```python
from build123d import *

# Parameters (mm, degrees)
ESQUISSE1_W                                        = 10
ESQUISSE1_H                                        = 10
BOSS_EXTRU_1_DEPTH                                 = 58
ENL_V_MAT_EXTRU_2_REACH                            = 61.068
ESQUISSE12_R                                       = 3
CHANFREIN1_SIZE                                    = 0.2
CONG_1_R                                           = 2
TROU_TARAUD_M41_D                                  = 3.3
TROU_TARAUD_M41_DEPTH                              = 11.5
TROU_TARAUD_M41_TIP                                = 0.991420021
TROU_TARAUD_M42_D                                  = 3.3
TROU_TARAUD_M42_DEPTH                              = 11.5
TROU_TARAUD_M42_TIP                                = 0.991420021
DIAM_TRE_DU_PER_AGE_4_0_4_1_D                      = 4
DIAM_TRE_DU_PER_AGE_4_0_4_1_DEPTH                  = 5
DIAM_TRE_DU_PER_AGE_4_0_4_1_TIP                    = 1.201721238
CHAMBRAGE_POUR_VIS_T_TE_HEXAGONALE_M41_D           = 4.3
CHAMBRAGE_POUR_VIS_T_TE_HEXAGONALE_M41_CBORE_D     = 8
CHAMBRAGE_POUR_VIS_T_TE_HEXAGONALE_M41_CBORE_DEPTH = 4.4
TROU_TARAUD_M31_D                                  = 2.5
TROU_TARAUD_M31_DEPTH                              = 8.5
TROU_TARAUD_M31_TIP                                = 0.751075774
ESQUISSE25_W                                       = 10
ESQUISSE25_H                                       = 20
ENL_V_MAT_EXTRU_4_DEPTH                            = 3
CASSER_START                                       = -10
ESQUISSE26_W                                       = 5
ESQUISSE26_H                                       = 5
CASSER_ANGLE_DEPTH                                 = 10


with BuildPart() as part:
    # Esquisse1 → Boss.-Extru.1 (new, symmetric)
    with BuildSketch(Plane.XY):
        Rectangle(ESQUISSE1_W, ESQUISSE1_H)
    extrude(amount=BOSS_EXTRU_1_DEPTH, both=True)

    # Esquisse12 → Enlèv. mat.-Extru.2 (cut, up to next)
    with BuildSketch(Plane(origin=(0, 5, 0), x_dir=(1, 0, 0), z_dir=(0, 1, 0)), mode=Mode.PRIVATE) as enl_v_mat_extru_2_sk1:
        with Locations(Location((0, 0, 0), (0, 0, 180))):
            Circle(ESQUISSE12_R)
    enl_v_mat_extru_2_tool1 = extrude(enl_v_mat_extru_2_sk1.sketch, amount=-ENL_V_MAT_EXTRU_2_REACH, mode=Mode.PRIVATE) & part.part
    add(enl_v_mat_extru_2_tool1.solids().sort_by_distance((0, 5, 0))[0], mode=Mode.SUBTRACT)

    # Chanfrein1
    chanfrein1_edges = [part.edges().sort_by_distance(p)[0] for p in [
        (3, 5, 0),
        (3, -5, 0),
    ]]
    chamfer(chanfrein1_edges, length=CHANFREIN1_SIZE)

    # Congé1
    # the kernel refuses this fillet: 2 mm, written as the material it takes off along each edge
    with BuildSketch(Plane(origin=(-5, 5, -63), x_dir=(1, 0, 0), z_dir=(0, 0, 1)), Plane(origin=(5, 5, 63), x_dir=(-1, 0, 0), z_dir=(0, 0, -1)), Plane(origin=(5, -5, 63), x_dir=(0, 1, 0), z_dir=(0, 0, -1)), Plane(origin=(-5, -5, -63), x_dir=(0, 1, 0), z_dir=(0, 0, 1))) as cong_1_piece_1:
        with BuildLine():
            CenterArc((CONG_1_R, -CONG_1_R), CONG_1_R, 90, 90)
            Line((0, -CONG_1_R), (0, 0))
            Line((0, 0), (CONG_1_R, 0))
        make_face()
    extrude(amount=126, mode=Mode.SUBTRACT)

    # Trou taraudé M41
    with Locations(Plane.XY.offset(58)):
        with Locations((0, 0)):
            Hole(TROU_TARAUD_M41_D / 2, depth=TROU_TARAUD_M41_DEPTH)
            with Locations((0, 0, -(TROU_TARAUD_M41_DEPTH + TROU_TARAUD_M41_TIP / 2))):  # 118° drill point
                Cone(0, TROU_TARAUD_M41_D / 2, TROU_TARAUD_M41_TIP, mode=Mode.SUBTRACT)

    # Trou taraudé M42
    with Locations(Plane(origin=(0, 0, -58), x_dir=(-1, 0, 0), z_dir=(0, 0, -1))):
        with Locations((0, 0)):
            Hole(TROU_TARAUD_M42_D / 2, depth=TROU_TARAUD_M42_DEPTH)
            with Locations((0, 0, -(TROU_TARAUD_M42_DEPTH + TROU_TARAUD_M42_TIP / 2))):  # 118° drill point
                Cone(0, TROU_TARAUD_M42_D / 2, TROU_TARAUD_M42_TIP, mode=Mode.SUBTRACT)

    # Diamètre du perçage Ø4.0 (4)1
    with Locations(Plane(origin=(5, 0, 0), x_dir=(0, 0, -1), z_dir=(1, 0, 0))):
        with Locations((8, 0), (-8, 0)):
            Hole(DIAM_TRE_DU_PER_AGE_4_0_4_1_D / 2, depth=DIAM_TRE_DU_PER_AGE_4_0_4_1_DEPTH)
            with Locations((0, 0, -(DIAM_TRE_DU_PER_AGE_4_0_4_1_DEPTH + DIAM_TRE_DU_PER_AGE_4_0_4_1_TIP / 2))):  # 118° drill point
                Cone(0, DIAM_TRE_DU_PER_AGE_4_0_4_1_D / 2, DIAM_TRE_DU_PER_AGE_4_0_4_1_TIP, mode=Mode.SUBTRACT)

    # Chambrage pour vis à tête hexagonale M41 (through all)
    with Locations(Plane.ZY.offset(5)):
        with Locations((-16, 0), (16, 0)):
            CounterBoreHole(CHAMBRAGE_POUR_VIS_T_TE_HEXAGONALE_M41_D / 2, CHAMBRAGE_POUR_VIS_T_TE_HEXAGONALE_M41_CBORE_D / 2, CHAMBRAGE_POUR_VIS_T_TE_HEXAGONALE_M41_CBORE_DEPTH)

    # Trou taraudé M31
    with Locations(Plane.ZY.offset(5)):
        with Locations((-8, 0), (8, 0)):
            Hole(TROU_TARAUD_M31_D / 2, depth=TROU_TARAUD_M31_DEPTH)
            with Locations((0, 0, -(TROU_TARAUD_M31_DEPTH + TROU_TARAUD_M31_TIP / 2))):  # 118° drill point
                Cone(0, TROU_TARAUD_M31_D / 2, TROU_TARAUD_M31_TIP, mode=Mode.SUBTRACT)

    # Esquisse25 → Enlèv. mat.-Extru.4 (cut)
    with BuildSketch(Plane.ZY.offset(5)):
        Rectangle(ESQUISSE25_W, ESQUISSE25_H)
    extrude(amount=-ENL_V_MAT_EXTRU_4_DEPTH, mode=Mode.SUBTRACT)

    # Esquisse26 → Casser Angle (cut)
    with BuildSketch(Plane(origin=(0, 5, 0), x_dir=(1, 0, 0), z_dir=(0, 1, 0)).offset(CASSER_START)):
        with Locations((-2.5, 0)):
            Rectangle(ESQUISSE26_W, ESQUISSE26_H)
    extrude(amount=CASSER_ANGLE_DEPTH, mode=Mode.SUBTRACT)


solid = part.part
```
The listing builds one solid part. Answer for the finished solid, in the listing's coordinates (mm). A direction names the side the tool comes from. Give positions to 0.01 mm unless a question says otherwise; leave off trailing zeros. Order: outer loops, then holes, each group sorted by start corner. A loop starts at its lowest first (then second) coordinate and runs counter-clockwise, first axis right, second up. Notation, with made-up numbers: (2.25, -24.75) -> (32.25, -24.75) arc R30 cw to (32.25, 1.25) -> close; hole circle Ø2 at (56.5, 34.25). An arc over 180 degrees is marked (long way). Write each question's results on one line, items separated by ' | '.
Q1. Determine the mould class of faces 1 (the face through (-4.4, 4.43, 31.13)), 2 (the face through (3, 0, 0)), 3 (the face through (2, 0, -58)), 4 (the face through (-2.831, -1.532, -12.305)) for opening direction Z: pulls with the +Z half, pulls with the -Z half, needs draft (parallel to the pull), parting line crosses it, or undercut.
Checked values:
face 1: needs draft | face 2: undercut | face 3: pulls with the -Z half | face 4: undercut
Q2. Which of the six approach directions +Z, -Z, +X, -X, +Y, -Y give full straight-line access (tool end or side, diameter ignored) to faces 5 (the face through (-2.831, 1.201, 19.815)), 6 (the face through (2.5, -1.2, -9.6)), 7 (the face through (-2, 0, -4)), 8 (the face through (-4.43, -4.4, -31.87))?
Checked values:
face 5: -X | face 6: +X | face 7: -X, +Y, -Y | face 8: +Z, -Z, -X, -Y
Q3. The part is cut by section B-B, the plane z = -28. Give the vertices of the cut face in (x, y).
Checked values:
outline: (-5, -3) arc R2 ccw to (-3, -5) -> (3, -5) arc R2 ccw to (5, -3) -> (5, 3) arc R2 ccw to (3, 5) -> (-3, 5) arc R2 ccw to (-5, 3) -> close
Q4. Each of these flat-tipped pins is pushed along its axis until it touches: P1, Ø3.5, axis at x = 0, z = 0, coming from the +Y side; P2, Ø1, axis at y = 3.5, z = -39.5, coming from the +X side; P3, Ø3, axis at x = 0, y = 0, coming from the +Z side; P4, Ø3, axis at y = 0, z = 8, coming from the +X side. Where does it stop, or does it pass through?
Checked values:
P1: passes through | P2: stops at x = 5 | P3: stops at z = 46.41 | P4: stops at x = -0.3
Q5. Straight lines are drawn through the part: probe 1 along Z at (x, y) = (-1.75, 0); probe 2 along Z at (x, y) = (2.25, -3); probe 3 along Z at (x, y) = (-0.5, -0.75). For each, find the intervals that lie inside material, in ascending order. Write a range as from..to.
Checked values:
probe 1: z = -58..-20, -12..-9.25, -6.75..-2.5, 2.5..6.75, 9.25..12, 20..58 | probe 2: z = -58..-1.98, 1.98..58 | probe 3: z = -46.05..-18.01, -13.99..-9, -7..-2.96, 2.96..7, 9..13.99, 18.01..46.05
Q6. The part is cut by section A-A, the plane z = -8. Give the vertices of the cut face in (x, y), and give its area (3 significant figures).
Checked values:
outline: (-5, -3) arc R2 ccw to (-3, -5) -> (3, -5) arc R2 ccw to (5, -3) -> (5, -2) -> (0, -2) -> (-0.45, -1.25) -> (-5, -1.25) -> close; (-5, 1.25) -> (-0.45, 1.25) -> (0, 2) -> (5, 2) -> (5, 3) arc R2 ccw to (3, 5) -> (-3, 5) arc R2 ccw to (-5, 3) -> close | area: 63.7 mm^2
